from build123d import *

# Parameters (mm, degrees)
F1_DEPTH = 12.7
F2_DEPTH = 12.7
F4_COUNT = 10


with BuildPart() as f1:
    # F0 (on Front) → F1 (new body)
    with BuildSketch(Plane.XZ):
        with BuildLine():
            ThreePointArc((-18.2398537228, 47.4125272072), (-28.7580895652, -41.8761541281), (50.8, 0))
            ThreePointArc((50.8, 0), (37.6668973466, 34.0858452188), (5.0580769968, 50.5475603476))
            ThreePointArc((5.0580769968, 50.5475603476), (-6.7747263864, 50.3462320575), (-18.2398537228, 47.4125272072))
        make_face()
    extrude(amount=F1_DEPTH)

    # F0 (on Front) → F2 (join, through all)
    with BuildSketch(Plane.XZ):
        with BuildLine():
            ThreePointArc((-18.2398537228, 47.4125272072), (-6.7747263864, 50.3462320575), (5.0580769968, 50.5475603476))
            add(Edge.make_bspline(
                [(5.0580769968, 50.5475603476), (4.8787158838, 52.5914812168), (4.4897162166, 56.9263105927), (0.1861426341, 63.9548196192), (-4.9903423699, 68.7921425636), (-7.7980468665, 71.4175781238)],
                knots=[0, 0, 0, 0, 0.2880613085, 0.6141610371, 1, 1, 1, 1], degree=3))
            Line((-7.7980468665, 71.4175781238), (-11.3577849389, 70.9385700538))
            add(Edge.make_bspline(
                [(-18.2398537228, 47.4125272072), (-18.6071605924, 49.4311575825), (-19.3778623389, 53.7146240849), (-17.0852769639, 61.6307302623), (-13.371613766, 67.6643358111), (-11.3577849389, 70.9385700538)],
                knots=[0, 0, 0, 0, 0.2880613085, 0.6141610371, 1, 1, 1, 1], degree=3))
        make_face()
    extrude(amount=F2_DEPTH)

    # F4: F1 ×10 about axis
    f4_axis = Axis((0, -10.3239128366, 0), (0, -1, 0))


with BuildPart() as f1_1:
    add(f1.part)
    for i in range(1, F4_COUNT):
        add(f1.part.rotate(f4_axis, i * 360 / F4_COUNT))


solid = f1_1.part
Input: part model. Units: mm. Frame: model coordinates. A direction names the side the tool comes from. Round coordinates to 2 decimals unless told otherwise and drop trailing zeros. Answer as a JSON object with one key per item and string values. Group by question number.
(1) Draft query along Z for faces 1 (the face through (9.55, -6.26, -71.18)), 2 (the face through (34.111, -6.261, 63.202)), 3 (the face through (-44.686, -6.261, 24.162)), 4 (the face through (50.354, -6.261, 6.718)). Return one class per face: released by +Z, released by -Z, zero draft, split by the parting line, or undercut.
(2) Reachability of faces 5 (the face through (-9.171, -6.261, -49.965)), 6 (the face through (36.79, -6.26, 35.03)), 7 (the face through (64.746, -6.261, 31.082)), 8 (the face through (9.171, -6.261, 49.965)), 9 (the face through (-70.65, -6.26, 12.91)) from +Z, -Z, +X, -X, +Y, -Y: full face, straight path, thin tool, end or side. Return the list, or none.
(3) Pin query (flat end, axial travel): P1, Ø6, axis at y = -6, z = 21.5, coming from the -X side; P2, Ø3, axis at y = -6.5, z = 15.5, coming from the -X side; P3, Ø4, axis at y = -3, z = -7, coming from the -X side; P4, Ø2, axis at x = 9, z = -18, coming from the +Y side. Return the tip coordinate at first contact, or that it passes through.
(4) Material intervals for probe 1 along X at (y, z) = (-2, -64); probe 2 along Z at (x, y) = (54, -10); probe 3 along X at (y, z) = (-6, 56), sorted ascending. Write a range as from..to.
Here are the results:
{
 "1": {"face 1": "released by -Z", "face 2": "released by +Z", "face 3": "undercut", "face 4": "undercut"},
 "2": {"face 5": "-Z, +Y, -Y", "face 6": "+Y, -Y", "face 7": "+Z, +X, +Y, -Y", "face 8": "+Z, +Y, -Y", "face 9": "+Z, -X, +Y, -Y"},
 "3": {"P1": "stops at x = -63", "P2": "stops at x = -70.45", "P3": "stops at x = -50.55", "P4": "stops at y = 0"},
 "4": {"probe 1": "x = -32.63..-32.35, 0.42..15.43", "probe 2": "z = -21.26..2.17, 12.93..34.78", "probe 3": "x = -18.53..4.22, 17.71..36.81"}
}
